```python
from build123d import *

# Parameters (mm, degrees)
SKETCH1_R           = 62.5
BOSS_EXTRUDE1_DEPTH = 21
SKETCH2_R           = 32
SKETCH2_R_2         = 6
CUT_EXTRUDE1_DEPTH  = 16
SKETCH3_R           = 6
SKETCH3_R_2         = 4
CUT_EXTRUDE2_DEPTH  = 14
CUT_EXTRUDE7_START  = -5
CUT_EXTRUDE7_DEPTH  = 5
FILLET1_R           = 1.5
BOSS_EXTRUDE2_START = 1
SKETCH12_R          = 4
BOSS_EXTRUDE2_DEPTH = 1
BOSS_EXTRUDE3_DEPTH = 1
SKETCH14_W          = 5
SKETCH14_H          = 8
CUT_EXTRUDE9_DEPTH  = 5


# Read off the part's stored shape, not the designer's step: Cut-Extrude7
with BuildPart() as part:
    # Sketch1 → Boss-Extrude1 (new body)
    with BuildSketch(Plane(origin=(0, 0, 0), x_dir=(1, 0, 0), z_dir=(0, 1, 0))):
        with Locations(Location((0, 0, 0), (0, 0, 90))):
            Circle(SKETCH1_R)
    extrude(amount=BOSS_EXTRUDE1_DEPTH)

    # Sketch2 → Cut-Extrude1 (cut)
    with BuildSketch(Plane(origin=(0, 21, 0), x_dir=(1, 0, 0), z_dir=(0, 1, 0))):
        with Locations(Location((0, 0, 0), (0, 0, 270))):
            Circle(SKETCH2_R)
        with Locations(Location((0, 0, 0), (0, 0, 270))):
            Circle(SKETCH2_R_2, mode=Mode.SUBTRACT)
    extrude(amount=-CUT_EXTRUDE1_DEPTH, mode=Mode.SUBTRACT)

    # Sketch3 → Cut-Extrude2 (cut)
    with BuildSketch(Plane(origin=(0, 21, 0), x_dir=(1, 0, 0), z_dir=(0, 1, 0))):
        with Locations(Location((0, 0, 0), (0, 0, 270))):
            Circle(SKETCH3_R)
        with Locations(Location((0, 0, 0), (0, 0, 270))):
            Circle(SKETCH3_R_2, mode=Mode.SUBTRACT)
    extrude(amount=-CUT_EXTRUDE2_DEPTH, mode=Mode.SUBTRACT)

    # Cut-Extrude7 outline → Cut-Extrude7 (cut)
    with BuildSketch(Plane(origin=(0, 21, 0), x_dir=(1, 0, 0), z_dir=(0, 1, 0)).offset(CUT_EXTRUDE7_START)):
        with BuildLine():
            Line((-48.023431781, -40), (11.976568219, -40))
            Line((11.976568219, -40), (11.976568219, -35))
            Line((11.976568219, -35), (-51.780787943, -35))
            ThreePointArc((-51.780787943, -35), (-49.964693221, -37.547029594), (-48.023431781, -40))
        make_face()
        with BuildLine():
            Line((-6.031762045, -54), (31.468237955, -54))
            ThreePointArc((31.468237955, -54), (34.542067999, -52.087383677), (37.5, -50))
            Line((37.5, -50), (-6.031762045, -50))
            Line((-6.031762045, -50), (-6.031762045, -54))
        make_face()
        with BuildLine():
            ThreePointArc((40.620192023, -47.5), (43.295213632, -45.075209113), (45.82575695, -42.5))
            Line((45.82575695, -42.5), (-19.379807977, -42.5))
            Line((-19.379807977, -42.5), (-19.379807977, -47.5))
            Line((-19.379807977, -47.5), (40.620192023, -47.5))
        make_face()
        with BuildLine():
            ThreePointArc((-17.5, -26.790856649), (-20.101587243, -24.898317018), (-22.5, -22.754120506))
            Line((-22.5, -22.754120506), (-22.5, -30.05))
            Line((-22.5, -30.05), (-17.5, -30.05))
            Line((-17.5, -30.05), (-17.5, -26.790856649))
        make_face()
        with BuildLine():
            Line((-22.5, 30.05), (-22.5, 22.754120506))
            ThreePointArc((-22.5, 22.754120506), (-20.101587243, 24.898317018), (-17.5, 26.790856649))
            Line((-17.5, 26.790856649), (-17.5, 30.05))
            Line((-17.5, 30.05), (-22.5, 30.05))
        make_face()
        with BuildLine():
            ThreePointArc((22.5, -22.754120506), (20.101587243, -24.898317018), (17.5, -26.790856649))
            Line((17.5, -26.790856649), (17.5, -30.05))
            Line((17.5, -30.05), (22.5, -30.05))
            Line((22.5, -30.05), (22.5, -22.754120506))
        make_face()
        with BuildLine():
            Line((17.5, 30.05), (17.5, 26.790856649))
            ThreePointArc((17.5, 26.790856649), (20.101587243, 24.898317018), (22.5, 22.754120506))
            Line((22.5, 22.754120506), (22.5, 30.05))
            Line((22.5, 30.05), (17.5, 30.05))
        make_face()
    extrude(amount=CUT_EXTRUDE7_DEPTH, mode=Mode.SUBTRACT)

    # Fillet1
    fillet1_edges = [part.edges().sort_by_distance(p)[0] for p in [
        (-10.840600106, 21, 61.552671667),
        (39.080092124, 21, 48.774956684),
        (57.282196187, 21, -25),
    ]]
    fillet(fillet1_edges, radius=FILLET1_R)

    # Sketch12 → Boss-Extrude2 (add)
    with BuildSketch(Plane(origin=(0, 21, 0), x_dir=(1, 0, 0), z_dir=(0, 1, 0)).offset(BOSS_EXTRUDE2_START)):
        with Locations(Location((0, 0, 0), (0, 0, 270))):
            Circle(SKETCH12_R)
    extrude(amount=-BOSS_EXTRUDE2_DEPTH)

    # Sketch13 → Boss-Extrude3 (add)
    with BuildSketch(Plane(origin=(0, 21, 0), x_dir=(1, 0, 0), z_dir=(0, 1, 0))):
        with BuildLine():
            Line((-3.75, -3.142053469), (3.75, -3.142053469))
            ThreePointArc((3.75, -3.142053469), (4.892340953, 0), (3.75, 3.142053469))
            Line((3.75, 3.142053469), (-3.75, 3.142053469))
            ThreePointArc((-3.75, 3.142053469), (-4.892340953, 0), (-3.75, -3.142053469))
        make_face()
    extrude(amount=BOSS_EXTRUDE3_DEPTH)

    # Sketch14 → Cut-Extrude9 (cut)
    with BuildSketch(Plane(origin=(0, 22, 0), x_dir=(1, 0, 0), z_dir=(0, 1, 0))):
        Rectangle(SKETCH14_W, SKETCH14_H)
    extrude(amount=-CUT_EXTRUDE9_DEPTH, mode=Mode.SUBTRACT)

    # Sketch16 → Cut-Revolve1 (revolve, cut)
    with BuildSketch(Plane.XY, mode=Mode.PRIVATE) as cut_revolve1_sk:
        Polygon((4.892340953, 21), (4, 22), (4.892340953, 22), align=None)
    revolve(cut_revolve1_sk.sketch.rotate(Axis((0, 0, 0), (0, 1, 0)), 214.055797743), axis=Axis((0, 0, 0), (0, 1, 0)), mode=Mode.SUBTRACT)


solid = part.part
```
Build history of the part. All positions in model axes, mm. A direction names the side the tool comes from. Coordinates: 2 decimals unless noted, no trailing zeros. Order: outer loops, then holes, each group sorted by start corner. A loop starts at its lowest first (then second) coordinate and runs counter-clockwise, first axis right, second up. Notation, with made-up numbers: (33.5, 48.25) -> (75.5, 48.25) arc R23 cw to (75.5, 86.25) -> close; hole circle Ø11 at (52.5, -16.5). An arc over 180 degrees is marked (long way). Answer in a Markdown table with one row per item. Add a question column.
Q1. Drop flat-ended pins along their axis: pin 1 (2.5 mm diameter, centred on y = 19, z = 28, fed in from -X); pin 2 (5.5 mm diameter, centred on y = 19.5, z = 37.5, fed in from -X); pin 3 (3 mm diameter, centred on x = -30, y = 3, fed in from -Z). Give the stop position or say it passes through.
Q2. Which spindle directions (+Z, -Z, +X, -X, +Y, -Y) get a long thin tool onto all of the face, cutting with end or side? Do faces 1 (the face through (-19.38, 18, 45)), 2 (the face through (-17.5, 18, -28)), 3 (the face through (11.977, 18, 38)). Say none if no direction does.
Q3. Band-saw the part on C-C, the plane y = 12.75. List the corners of the cut face in (x, z).
Q4. Band-saw the part on A-A, the plane z = 0. List the corners of the cut face in (x, y).
Q5. Wall check: line 1 along X through (y, z) = (10.25, 0); line 2 along X through (y, z) = (18.25, 0); line 3 along Y through (x, z) = (-45, 4). Give the ranges that are in metal, low to high. Write a range as [from, to].
Answers follow:
| question | item | result |
|---|---|---|
| 1 | pin 1 | x = -56.49 |
| 1 | pin 2 | x = -51.95 |
| 1 | pin 3 | z = -55.62 |
| 2 | face 1 | +X, +Y |
| 2 | face 2 | +Y |
| 2 | face 3 | -X, +Y |
| 3 | outline | circle Ø125 at (0, 0); circle Ø8 at (0, 0); hole circle Ø64 at (0, 0) |
| 4 | outline | (-62.5, 0) -> (62.5, 0) -> (62.5, 19.5) arc R1.5 ccw to (61, 21) -> (32, 21) -> (32, 5) -> (6, 5) -> (6, 7) -> (4, 7) -> (4, 21) -> (4.89, 21) -> (4, 22) -> (2.5, 22) -> (2.5, 17) -> (-2.5, 17) -> (-2.5, 22) -> (-4, 22) -> (-4.89, 21) -> (-4, 21) -> (-4, 7) -> (-6, 7) -> (-6, 5) -> (-32, 5) -> (-32, 21) -> (-61, 21) arc R1.5 ccw to (-62.5, 19.5) -> close |
| 5 | line 1 | [-62.5, -32], [-4, 4], [32, 62.5] |
| 5 | line 2 | [-62.5, -32], [-4, -2.5], [2.5, 4], [32, 62.5] |
| 5 | line 3 | [0, 21] |
